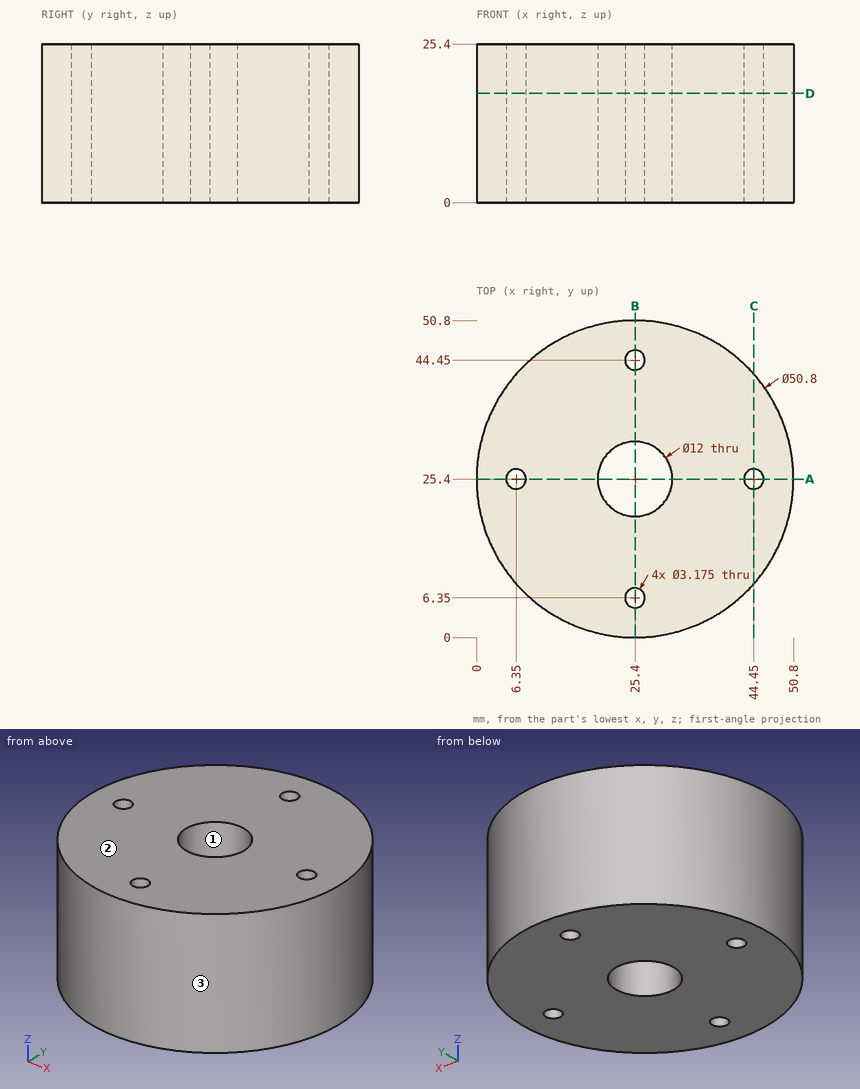
The drawing under review shows one solid part. Ordinate dimensions are in mm from its lowest x, y, z. Round coordinates to 2 decimals unless told otherwise and drop trailing zeros. Order: outer loops, then holes, each group sorted by start corner. A loop starts at its lowest first (then second) coordinate and runs counter-clockwise, first axis right, second up. Notation, with made-up numbers: (84, 27) -> (95, 27) arc R19 ccw to (95, 50) -> close; hole circle Ø2 at (3, -30). An arc over 180 degrees is marked (long way). Return JSON: item names as keys, results as strings.
1. Take a section at A-A (y = 25.4). Write out the cut boundary in (x, z).
Answer block:
{"outline": "(0, 0) -> (4.76, 0) -> (4.76, 25.4) -> (0, 25.4) -> close; (7.94, 0) -> (19.4, 0) -> (19.4, 25.4) -> (7.94, 25.4) -> close; (31.4, 0) -> (42.86, 0) -> (42.86, 25.4) -> (31.4, 25.4) -> close; (46.04, 0) -> (50.8, 0) -> (50.8, 25.4) -> (46.04, 25.4) -> close"}
2. Insertion check: P1, Ø2.5, axis at x = 44.45, y = 25.4, coming from the +Z side; P2, Ø4, axis at x = 11, y = 21, coming from the -Z side; P3, Ø3, axis at x = 41.5, z = 7, coming from the -Y side; P4, Ø10, axis at y = 41, z = 8, coming from the +X side. Each pin has a flat end and moves straight along its axis. Give the tip position at first contact, or say it passes through.
Answer block:
{"P1": "passes through", "P2": "stops at z = 0", "P3": "stops at y = 4.62", "P4": "stops at x = 48.48"}
3. Take a section at D-D (z = 17.5). State how many separate pieces and enclosed holes the cut face has, then the cut area to 3 significant figures.
Answer block:
{"separate pieces": "1", "enclosed holes": "5", "area": "1,880 mm²"}
4. The part is to be moulded in two halves that separate along Y. For the marked faces 1, 2 and 3, say which applies: +Y half, -Y half, draft (parallel to the pull), parting line (faces both ways), or undercut.
Answer block:
{"face 1": "undercut", "face 2": "draft", "face 3": "parting line"}
5. For L1, parallel to Y at x = 25.4, z = 11; L2, parallel to X at y = 5.5, z = 16.25; L3, parallel to X at y = 6, z = 1, list the stretches that pass through material, from the lowest coordinate up. Write a range as [from, to].
Answer block:
{"L1": "y = [0, 4.76], [7.94, 19.4], [31.4, 42.86], [46.04, 50.8]", "L2": "x = [9.62, 24.06], [26.74, 41.18]", "L3": "x = [9, 23.85], [26.95, 41.8]"}
6. Take a section at C-C (x = 44.45). Write out the cut boundary in (y, z).
Answer block:
{"outline": "(8.6, 0) -> (23.81, 0) -> (23.81, 25.4) -> (8.6, 25.4) -> close; (26.99, 0) -> (42.2, 0) -> (42.2, 25.4) -> (26.99, 25.4) -> close"}
